Read the model definition and answer for the solid it produces. Units are mm, in the model's axes. Face numbers are marked on the shaded views. A direction names the side the tool comes from. Round coordinates to 2 decimals unless told otherwise and drop trailing zeros. Write each loop counter-clockwise with the first axis right and the second up, starting at its lowest first coordinate (ties: lowest second). Pieces come first, ordered by that corner, then holes. Notation, with made-up numbers: (86, -30.75) -> (138, -30.75) arc R20 ccw to (138, 7.25) -> close; hole circle Ø5 at (48, 48.5). An arc over 180 degrees is marked (long way). Return JSON: item names as keys, results as strings.
from build123d import *

# Parameters (mm, degrees)
SKETCH1_R           = 2.75
SKETCH1_R_2         = 12.1
BOSS_EXTRUDE1_DEPTH = 8
SKETCH3_R           = 2.75
SKETCH3_R_2         = 5
BOSS_EXTRUDE3_DEPTH = 2
BOSS_EXTRUDE4_DEPTH = 15
FILLET1_R           = 10
SKETCH5_R           = 2.85
CUT_EXTRUDE1_DEPTH  = 40
BOSS_EXTRUDE5_DEPTH = 5
CHAMFER1_SIZE       = 2.5


with BuildPart() as part:
    # Sketch1 → Boss-Extrude1 (new body)
    with BuildSketch(Plane(origin=(0, 0, 0), x_dir=(1, 0, 0), z_dir=(0, 1, 0))):
        with BuildLine():
            Line((-20, 0), (20, 0))
            Line((20, 0), (20, 85))
            ThreePointArc((20, 85), (0, 105), (-20, 85))
            Line((-20, 85), (-20, 0))
        make_face()
        with Locations(Location((0, 10, 0), (0, 0, 270))):
            Circle(SKETCH1_R, mode=Mode.SUBTRACT)
        with Locations(Location((0, 82, 0), (0, 0, 270))):
            Circle(SKETCH1_R_2, mode=Mode.SUBTRACT)
        with Locations(Location((0, 35, 0), (0, 0, 270))):
            Circle(SKETCH1_R, mode=Mode.SUBTRACT)
    extrude(amount=BOSS_EXTRUDE1_DEPTH)

    # Sketch3 → Boss-Extrude3 (add)
    with BuildSketch(Plane(origin=(0, 8, 0), x_dir=(1, 0, 0), z_dir=(0, 1, 0))):
        with BuildLine():
            Line((-20, 0), (20, 0))
            Line((20, 0), (20, 85))
            ThreePointArc((20, 85), (0, 105), (-20, 85))
            Line((-20, 85), (-20, 0))
        make_face()
        with Locations(Location((0, 10, 0), (0, 0, 270))):
            Circle(SKETCH3_R, mode=Mode.SUBTRACT)
        with Locations(Location((0, 35, 0), (0, 0, 270))):
            Circle(SKETCH3_R, mode=Mode.SUBTRACT)
        with Locations(Location((0, 82, 0), (0, 0, 270))):
            Circle(SKETCH3_R_2, mode=Mode.SUBTRACT)
    extrude(amount=BOSS_EXTRUDE3_DEPTH)

    # Sketch4 → Boss-Extrude4 (add, symmetric)
    with BuildSketch(Plane.XY.offset(-30)):
        Polygon((20, 0), (105, 0), (105, 40), (95, 40), (95, 13.535533906), (91.464466094, 10), (20, 10), align=None)
    extrude(amount=BOSS_EXTRUDE4_DEPTH, both=True)

    # Fillet1
    fillet1_edges = [part.edges().sort_by_distance(p)[0] for p in [
        (20, 5, -45),
        (20, 5, -15),
    ]]
    fillet(fillet1_edges, radius=FILLET1_R)

    # Sketch5 → Cut-Extrude1 (cut)
    with BuildSketch(Plane(origin=(105, 0, 0), x_dir=(0, 0, -1), z_dir=(1, 0, 0))):
        with Locations(Location((30, 25, 0), (0, 0, 90))):
            Circle(SKETCH5_R)
    extrude(amount=-CUT_EXTRUDE1_DEPTH, mode=Mode.SUBTRACT)

    # Sketch6 → Boss-Extrude5 (add)
    with BuildSketch(Plane.XY.offset(-15)):
        Polygon((65, 10), (95, 10), (95, 40), align=None)
    boss_extrude5 = extrude(amount=-BOSS_EXTRUDE5_DEPTH)

    # Mirror1: Boss-Extrude5 across plane
    add(boss_extrude5.mirror(Plane.XY.offset(-30)))

    # Chamfer1
    chamfer1_edges = [part.edges().sort_by_distance(p)[0] for p in [
        (0, 10, -12.75),
        (0, 10, -37.75),
    ]]
    chamfer(chamfer1_edges, length=CHAMFER1_SIZE)


solid = part.part
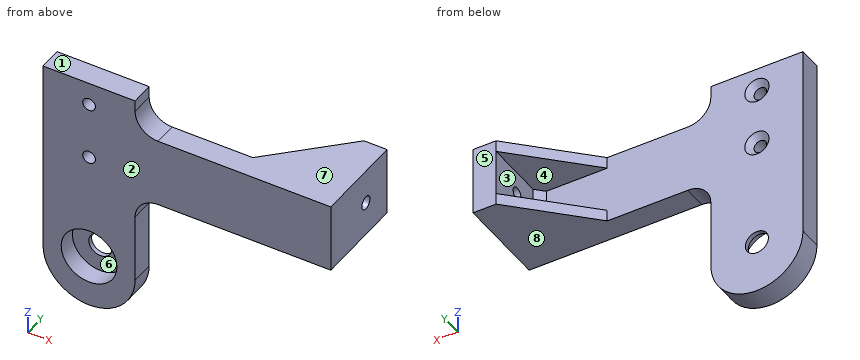
Item 1: A tool of negligible diameter and unlimited length cuts with its end or side. For the marked faces 4, 5, 6, 7 and 8, from which of +Z, -Z, +X, -X, +Y, -Y can it reach the whole face along a straight path? Write none if from no direction.
Worked answers:
{"face 4": "-X, +Y", "face 5": "+Z, -Z, +X, -X, +Y", "face 6": "-Y", "face 7": "+Z, +X, +Y, -Y", "face 8": "-Z, +X, +Y, -Y"}
Item 2: For a pull along Z with two mould halves and no side action, classify the marked faces 1, 2 and 3 as released by +Z, released by -Z, zero draft, split by the parting line, or undercut.
Worked answers:
{"face 1": "released by +Z", "face 2": "zero draft", "face 3": "undercut"}
Item 3: Flat-ended cylindrical pins translate along their axes: pin 1 (11 mm diameter, centred on y = 6, z = -70.5, fed in from +X); pin 2 (24 mm diameter, centred on x = 74, y = 20.5, fed in from -Z); pin 3 (10 mm diameter, centred on y = 25.5, z = -32, fed in from -X). Find the tip coordinate at first contact, or state that the pin passes through.
Worked answers:
{"pin 1": "stops at x = 20", "pin 2": "stops at z = -45", "pin 3": "stops at x = 95"}
Item 4: Straight lines are drawn through the part: L1, parallel to Z at x = 83, y = 27; L2, parallel to X at y = 4, z = -35; L3, parallel to Z at x = 99.5, y = 25. For each, find the intervals that lie inside material, in ascending order. Write a range as [from, to].
Worked answers:
{"L1": "z = [-45, -40], [-20, -15]", "L2": "x = [-20, -2.75], [2.75, 105]", "L3": "z = [-45, -32.85], [-27.15, -15]"}
Item 5: Section B-B (x = 81) is taken. Give the vertices of the cut face in (y, z), then the cut area to 3 significant figures.
Worked answers:
{"outline": "(0, -45) -> (26, -45) -> (26, -40) -> (10, -40) -> (10, -20) -> (26, -20) -> (26, -15) -> (0, -15) -> close", "area": "460 mm2"}
Item 6: Section A-A (y = 25) is taken. Give the vertices of the cut face in (x, z), then the cut area to 3 significant figures.
Worked answers:
{"outline": "(80, -45) -> (105, -45) -> (105, -32.85) -> (95, -32.85) -> (95, -40) -> (80, -40) -> close; (80, -20) -> (95, -20) -> (95, -27.15) -> (105, -27.15) -> (105, -15) -> (80, -15) -> close", "area": "393 mm2"}
Item 7: Section C-C (y = 17) is taken. Give the vertices of the cut face in (x, z).
Worked answers:
{"outline": "(72, -45) -> (105, -45) -> (105, -15) -> (72, -15) -> (72, -20) -> (95, -20) -> (95, -40) -> (72, -40) -> close"}
Item 8: Section D-D (z = -10) is taken. Give the vertices of the cut face in (x, y).
Worked answers:
{"outline": "(-20, 0) -> (-2.75, 0) -> (-2.75, 7.5) -> (-5.25, 10) -> (-20, 10) -> close; (2.75, 0) -> (21.34, 0) -> (21.34, 10) -> (5.25, 10) -> (2.75, 7.5) -> close"}
